```python
from build123d import *
from build123d.topology import SkipClean

# Parameters (mm, degrees)
CROQUIS1_R              = 15
SALIENTE_EXTRUIR1_DEPTH = 60
CROQUIS8_R              = 2.5
CORTAR_EXTRUIR2_DEPTH   = 15
SALIENTE_EXTRUIR3_START = 15
CROQUIS9_R              = 4
CROQUIS9_R_2            = 2.5
SALIENTE_EXTRUIR3_DEPTH = 7.5
CROQUIS10_R             = 4
SALIENTE_EXTRUIR4_DEPTH = 7.5
CROQUIS12_R             = 2.5
CORTAR_EXTRUIR4_DEPTH   = 30
CORTAR_EXTRUIR5_START   = 37.5
CROQUIS13_R             = 4
CORTAR_EXTRUIR5_DEPTH   = 30
CORTAR_EXTRUIR6_DEPTH   = 15
CROQUIS14_W             = 15
CROQUIS14_H             = 2.5
CORTAR_EXTRUIR7_DEPTH   = 4
CORTAR_EXTRUIR8_DEPTH   = 15
CROQUIS16_R             = 4
CORTAR_EXTRUIR9_DEPTH   = 7.5
CROQUIS17_W             = 15
CROQUIS17_H             = 4
CORTAR_EXTRUIR10_DEPTH  = 4


with BuildPart() as part:
    # Croquis1 → Saliente-Extruir1 (new body)
    with BuildSketch(Plane(origin=(0, 0, 0), x_dir=(1, 0, 0), z_dir=(0, 1, 0))):
        with Locations(Location((0, 0, 0), (0, 0, 270))):
            Circle(CROQUIS1_R)
    extrude(amount=SALIENTE_EXTRUIR1_DEPTH)

    # Croquis8 → Cortar-Extruir2 (cut, symmetric)
    with BuildSketch(Plane.XY):
        with Locations((0, 60)):
            Circle(CROQUIS8_R)
    extrude(amount=CORTAR_EXTRUIR2_DEPTH, both=True, mode=Mode.SUBTRACT)

    # Croquis9 → Saliente-Extruir3 (add)
    with BuildSketch(Plane.XY.offset(SALIENTE_EXTRUIR3_START)):
        with Locations((0, 60)):
            Circle(CROQUIS9_R)
        with Locations((0, 60)):
            Circle(CROQUIS9_R_2, mode=Mode.SUBTRACT)
    saliente_extruir3 = extrude(amount=-SALIENTE_EXTRUIR3_DEPTH)

    # Simetr_a2: Saliente-Extruir3 across plane
    with SkipClean():  # the faces are left unmerged after this step: merging them gives an invalid solid
        add(saliente_extruir3.mirror(Plane.XY))

    # Croquis10 → Saliente-Extruir4 (add, symmetric)
    with SkipClean():  # the faces are left unmerged after this step: merging them gives an invalid solid
        with BuildSketch(Plane.XY):
            Circle(CROQUIS10_R)
        extrude(amount=SALIENTE_EXTRUIR4_DEPTH, both=True)

    # Croquis12 → Cortar-Extruir4 (cut, symmetric)
    with SkipClean():  # the faces are left unmerged after this step: merging them gives an invalid solid
        with BuildSketch(Plane.XY.offset(7.5)):
            Circle(CROQUIS12_R)
        extrude(amount=CORTAR_EXTRUIR4_DEPTH, both=True, mode=Mode.SUBTRACT)

    # Croquis13 → Cortar-Extruir5 (cut)
    with SkipClean():  # the faces are left unmerged after this step: merging them gives an invalid solid
        with BuildSketch(Plane.XY.offset(CORTAR_EXTRUIR5_START)):
            Circle(CROQUIS13_R)
        cortar_extruir5 = extrude(amount=-CORTAR_EXTRUIR5_DEPTH, mode=Mode.SUBTRACT)

    # Simetr_a3: Cortar-Extruir5 across plane
    with SkipClean():  # the faces are left unmerged after this step: merging them gives an invalid solid
        add(cortar_extruir5.mirror(Plane.XY), mode=Mode.SUBTRACT)

    # Croquis7 → Cortar-Extruir6 (cut, symmetric)
    with SkipClean():  # the faces are left unmerged after this step: merging them gives an invalid solid
        with BuildSketch(Plane.XY):
            Polygon((-4, 56.432940258), (-15, 46.623525966), (-15, 60), (-4, 60), align=None)
        cortar_extruir6 = extrude(amount=CORTAR_EXTRUIR6_DEPTH, both=True, mode=Mode.SUBTRACT)

    # Croquis14 → Cortar-Extruir7 (cut)
    with SkipClean():  # the faces are left unmerged after this step: merging them gives an invalid solid
        with BuildSketch(Plane.ZY.offset(4)):
            with Locations((0, 58.75)):
                Rectangle(CROQUIS14_W, CROQUIS14_H)
        extrude(amount=-CORTAR_EXTRUIR7_DEPTH, mode=Mode.SUBTRACT)

    # Simetr_a4: Cortar-Extruir6 across plane
    with SkipClean():  # the faces are left unmerged after this step: merging them gives an invalid solid
        add(cortar_extruir6.mirror(Plane.ZX.offset(30)), mode=Mode.SUBTRACT)

    # Croquis15 → Cortar-Extruir8 (cut, symmetric)
    with SkipClean():  # the faces are left unmerged after this step: merging them gives an invalid solid
        with BuildSketch(Plane.XY):
            with BuildLine():
                Line((0, 4), (-8.002010921, 4))
                Line((-8.002010921, 4), (-8.002010921, -4.658510033))
                Line((-8.002010921, -4.658510033), (0, -4.658510033))
                Line((0, -4.658510033), (0, -4))
                ThreePointArc((0, -4), (-4, 0), (0, 4))
            make_face()
        extrude(amount=CORTAR_EXTRUIR8_DEPTH, both=True, mode=Mode.SUBTRACT)

    # Croquis16 → Cortar-Extruir9 (cut, symmetric)
    with SkipClean():  # the faces are left unmerged after this step: merging them gives an invalid solid
        with BuildSketch(Plane.XY):
            with Locations((0, 60)):
                Circle(CROQUIS16_R)
        extrude(amount=CORTAR_EXTRUIR9_DEPTH, both=True, mode=Mode.SUBTRACT)

    # Croquis17 → Cortar-Extruir10 (cut)
    with SkipClean():  # the faces are left unmerged after this step: merging them gives an invalid solid
        with BuildSketch(Plane.ZY.offset(4)):
            with Locations((0, 58)):
                Rectangle(CROQUIS17_W, CROQUIS17_H)
        extrude(amount=-CORTAR_EXTRUIR10_DEPTH, mode=Mode.SUBTRACT)


solid = part.part
```
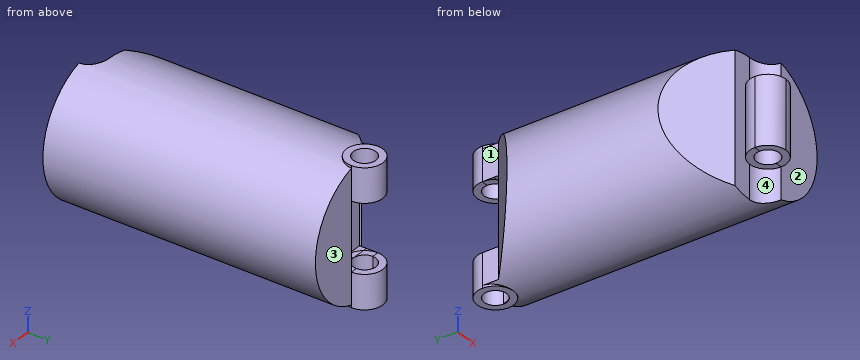
Could you check a few things on this model? Use its own coordinates, in mm. Face numbers are marked on the shaded views. A direction names the side the tool comes from. Coordinates: 2 decimals unless noted, no trailing zeros. Loops run counter-clockwise (first coordinate to the right, second up) from the corner with the lowest first, then second, coordinate; pieces in that order, holes last.
1) Imagine slicing it at B-B (x = 1). State how many separate pieces and enclosed holes the cut face has, and give its area (3 significant figures).
Reported:
separate pieces: 4
enclosed holes: 0
area: 1,660 mm2
2) Imagine slicing it at C-C (z = 10.5). List the corners of the cut face in (x, y) for me, and give its area (3 significant figures).
Reported:
outline: (-10.71, 9.55) - (-4.49, 4) - (0, 4) arc R4 cw to (4, 0) - (10.71, 0) - (10.71, 60) - (4, 60) arc R4 ccw to (-4, 60) - (-4, 56.43) - (-10.71, 50.45) - close; hole circle Ø5 at (0, 60)
area: 1,170 mm2
3) Imagine slicing it at D-D (x = -8). List the corners of the cut face in (y, z) for me, and give its area (3 significant figures).
Reported:
outline: (7.13, -12.69) - (52.87, -12.69) - (52.87, 12.69) - (7.13, 12.69) - close
area: 1,160 mm2
4) Please list where these lines run through material, in increasing order: line 1 along Z through (x, y) = (0.5, 57); line 2 along Y through (x, z) = (0, -12); line 3 along Z through (x, y) = (4, 59).
Reported:
line 1: z = -15 to -7.5, 7.5 to 15
line 2: y = 4 to 57.5, 62.5 to 64
line 3: z = -14.46 to 14.46
5) Will these pins go through, and if not, where does the flat tip stop? pin 1 Ø2 at (x, y) = (-0.5, -1) entering from +Z; pin 2 Ø12 at (x, z) = (9.5, -4) entering from -Y; pin 3 Ø2 at (x, z) = (-4.5, 10) entering from +Y; pin 4 Ø9 at (x, z) = (10.5, -6.5) entering from +Y.
Reported:
pin 1: passes through
pin 2: stops at y = -1.94
pin 3: stops at y = 61.94
pin 4: stops at y = 60
6) Which directions (+Z, -Z, +X, -X, +Y, -Y) give clear straight access to the entire face, cutting with the end or side of a thin tool? Please do the marked faces 1, 2, 3 and 4.
Reported:
face 1: +Z, -Z, -X, +Y
face 2: +Z, -Z, +X, -Y
face 3: +Z, -Z, +X, +Y
face 4: -Z, -X, -Y
7) Imagine slicing it at A-A (z = 0). List the corners of the cut face in (x, y) for me, and give its area (3 significant figures).
Reported:
outline: (-15, 13.38) - (-4.49, 4) - (0, 4) arc R4 ccw (long way) to (4, 0) - (15, 0) - (15, 60) - (4, 60) arc R4 cw to (0, 56) - (-4, 56) - (-4, 56.43) - (-15, 46.62) - close; hole circle Ø5 at (0, 0)
area: 1,590 mm2
